```python
from build123d import *

# Parameters (mm, degrees)
F1_DEPTH  = 16
F2_W      = 70
F2_H      = 3
F3_DEPTH  = 2
F4_W      = 50
F4_H      = 12
F5_DEPTH  = 2
F6_R      = 1
F9_DEPTH  = 2
F11_DEPTH = 38.001
F13_D     = 4
F14_R     = 3
F14_R_2   = 2
F15_DEPTH = 5


with BuildPart() as f1:
    # F0 (on Front) → F1 (new body)
    with BuildSketch(Plane.XZ):
        with BuildLine():
            Line((46.2855722755, 5.7414249778), (-47.7144277245, 5.7414249778))
            ThreePointArc((-47.7144277245, 5.7414249778), (-58.7144277245, -5.2585750222), (-47.7144277245, -16.2585750222))
            Line((-47.7144277245, -16.2585750222), (-28.7144277245, -16.2585750222))
            ThreePointArc((-28.7144277245, -16.2585750222), (-25.7968307423, -17.5210599177), (-24.7197856057, -20.5120821569))
            ThreePointArc((-24.7197856057, -20.5120821569), (-0.5386319719, -49.8206199667), (35.0020481502, -63.2585750222))
            ThreePointArc((35.0020481502, -63.2585750222), (39.8678360266, -64.6074545818), (44.1721712505, -67.2471640366))
            Line((44.1721712505, -67.2471640366), (45.9107602648, -66.2585750222))
            ThreePointArc((45.9107602648, -66.2585750222), (40.9429054682, -62.6971545828), (35.0020481502, -61.2585750222))
            ThreePointArc((35.0020481502, -61.2585750222), (0.6230450398, -48.7022972109), (-22.7197856057, -20.5120821569))
            ThreePointArc((-22.7197856057, -20.5120821569), (-24.3830859689, -16.1065299122), (-28.7144277245, -14.2585750222))
            Line((-28.7144277245, -14.2585750222), (-47.7144277245, -14.2585750222))
            ThreePointArc((-47.7144277245, -14.2585750222), (-56.7144277245, -5.2585750222), (-47.7144277245, 3.7414249778))
            Line((-47.7144277245, 3.7414249778), (46.2855722755, 3.7414249778))
            Line((46.2855722755, 3.7414249778), (46.2855722755, 5.7414249778))
        make_face()
    extrude(amount=F1_DEPTH)

    # F2 (on face) → F3 (join)
    with BuildSketch(Plane.XY.offset(5.7414249778)):
        with Locations((11.2855722755, -17.5)):
            Rectangle(F2_W, F2_H)
    extrude(amount=-F3_DEPTH)

    # F4 (on face) → F5 (join)
    with BuildSketch(Plane.XZ.offset(19)):
        with Locations((21.2855722755, -2.2585750222)):
            Rectangle(F4_W, F4_H)
    extrude(amount=-F5_DEPTH)

    # F6
    f6_edges = [f1.edges().sort_by_distance(p)[0] for p in [
        (11.285572, -19, 5.741425),
        (21.285572, -17, 3.741425),
    ]]
    fillet(f6_edges, radius=F6_R)

    # F7: F1 across plane


with BuildPart() as f1_1:
    add(f1.part)
    add(f1.part.mirror(Plane.XZ))

    # F8 (on face) → F9 (cut)
    with BuildSketch(Plane.XY.offset(5.7414249778)):
        with BuildLine():
            Line((46.2855722755, 12), (-13.7144277245, 12))
            ThreePointArc((-13.7144277245, 12), (-25.7144277245, 0), (-13.7144277245, -12))
            Line((-13.7144277245, -12), (46.2855722755, -12))
            Line((46.2855722755, -12), (46.2855722755, 12))
        make_face()
    extrude(amount=-F9_DEPTH, mode=Mode.SUBTRACT)

    # F10 (on face) → F11 (cut, through all)
    with BuildSketch(Plane.XZ.offset(19)):
        with BuildLine():
            ThreePointArc((2.2855722755, -0.2585750222), (-0.7144277245, -3.2585750222), (2.2855722755, -6.2585750222))
            Line((2.2855722755, -6.2585750222), (22.2855722755, -6.2585750222))
            ThreePointArc((22.2855722755, -6.2585750222), (25.2855722755, -3.2585750222), (22.2855722755, -0.2585750222))
            Line((22.2855722755, -0.2585750222), (2.2855722755, -0.2585750222))
        make_face()
    extrude(amount=-F11_DEPTH, mode=Mode.SUBTRACT)

    # F13 (through all)
    with Locations(Plane.XZ.offset(19)):
        with Locations((32.2855722755, -2.2585750222)):
            Hole(F13_D / 2)

    # F14 (on face) → F15 (join)
    with BuildSketch(Plane(origin=(0, -17, 0), x_dir=(-1, 0, 0), z_dir=(0, 1, 0))):
        with Locations((-32.2855722755, -2.2585750222)):
            Circle(F14_R)
        with Locations((-32.2855722755, -2.2585750222)):
            Circle(F14_R_2, mode=Mode.SUBTRACT)
    extrude(amount=F15_DEPTH)


solid = f1_1.part
```
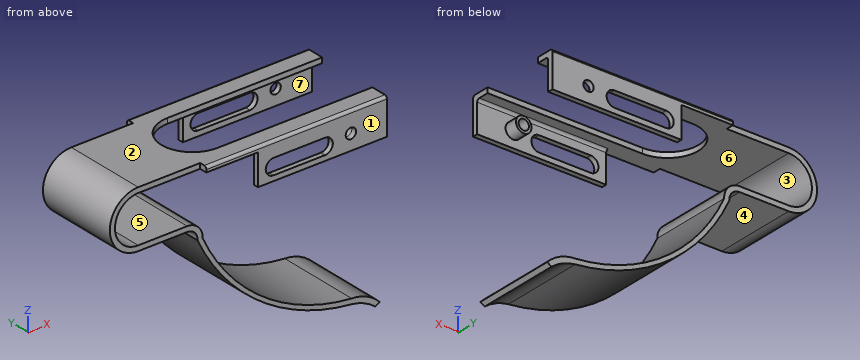
Design review of the part built by this model. Coordinates are the model's own, in mm. Face numbers are marked on the shaded views. A direction names the side the tool comes from. Round coordinates to 2 decimals unless told otherwise and drop trailing zeros. Write each loop counter-clockwise with the first axis right and the second up, starting at its lowest first coordinate (ties: lowest second). Pieces come first, ordered by that corner, then holes.
Item 1: For the marked faces 4, 5, 6 and 7, list the 3-axis set-ups (+Z, -Z, +X, -X, +Y, -Y) from which the entire face can be reached by the end or side of a thin tool; tool diameter is ignored.
Item 2: We need section D-D on z = -53.5. Write out the cut boundary in (x, y), and give its area (3 significant figures).
Item 3: We need section B-B on y = 0. Write out the cut boundary in (x, z).
Item 4: The part is to be moulded in two halves that separate along Z. For the marked faces 1, 2 and 3, say which applies: +Z half, -Z half, draft (parallel to the pull), parting line (faces both ways), or undercut.
Item 5: For probe 1 along X at (y, z) = (-13, -3); probe 2 along Z at (x, y) = (-53.5, -14.5); probe 3 along X at (y, z) = (2, -29.5), list the stretches that pass through material, from the lowest coordinate up.
Item 6: We need section A-A on x = -2.5. Write out the cut boundary in (y, z), and give its area (3 significant figures).
Item 7: Clearance check with flat-ended pins moving along their axes: pin 1 Ø1.6 at (x, y) = (10, 18) entering from -Z; pin 2 Ø0.6 at (y, z) = (17.5, 4.5) entering from -X; pin 3 Ø3 at (y, z) = (4.5, -49) entering from -X; pin 4 Ø3 at (x, z) = (32.29, -2.26) entering from -Y. State where each tip first meets the part, or that it passes through.
Item 8: We need section C-C on x = 24. Write out the cut boundary in (y, z), and give its area (3 significant figures).
Returned:
1. face 4: -Z, -X, +Y, -Y
1. face 5: +X, +Y, -Y
1. face 6: none
1. face 7: -Z, +X, -X
2. outline: (5.13, -16) - (8.47, -16) - (8.47, 16) - (5.13, 16) - close
2. area: 107 mm2
3. outline: (-47.71, -16.26) - (-28.71, -16.26) arc R4 cw to (-24.72, -20.51) arc R73.97 ccw to (35, -63.26) arc R18.11 cw to (44.17, -67.25) - (45.91, -66.26) arc R16 ccw to (35, -61.26) arc R70 cw to (-22.72, -20.51) arc R6 ccw to (-28.71, -14.26) - (-47.71, -14.26) arc R9 cw to (-47.71, 3.74) - (-25.71, 3.74) - (-25.71, 5.74) - (-47.71, 5.74) arc R11 ccw to start
4. face 1: draft
4. face 2: +Z half
4. face 3: undercut
5. probe 1: x = -58.48 to -56.43, 29.38 to 30.43, 34.14 to 35.19
5. probe 2: z = -14.61 to -12.15, 1.64 to 4.1
5. probe 3: x = -19.82 to -17.81
6. outline: (-19, -8.26) - (-17, -8.26) - (-17, 2.74) arc R1 cw to (-16, 3.74) - (-12, 3.74) - (-12, 5.74) - (-18, 5.74) arc R1 ccw to (-19, 4.74) - close; (-16, -48.37) - (16, -48.37) - (16, -46.36) - (-16, -46.36) - close; (12, 3.74) - (16, 3.74) arc R1 cw to (17, 2.74) - (17, -8.26) - (19, -8.26) - (19, 4.74) arc R1 ccw to (18, 5.74) - (12, 5.74) - close
6. area: 140 mm2
7. pin 1: stops at z = -8.26
7. pin 2: stops at x = -23.71
7. pin 3: stops at x = -3.61
7. pin 4: passes through
8. outline: (-19, -8.26) - (-17, -8.26) - (-17, -5.72) - (-19, -5.72) - close; (-19, -0.8) - (-17, -0.8) - (-17, 2.74) arc R1 cw to (-16, 3.74) - (-12, 3.74) - (-12, 5.74) - (-18, 5.74) arc R1 ccw to (-19, 4.74) - close; (-16, -61.29) - (16, -61.29) - (16, -59.42) - (-16, -59.42) - close; (12, 3.74) - (16, 3.74) arc R1 cw to (17, 2.74) - (17, -0.8) - (19, -0.8) - (19, 4.74) arc R1 ccw to (18, 5.74) - (12, 5.74) - close; (17, -8.26) - (19, -8.26) - (19, -5.72) - (17, -5.72) - close
8. area: 116 mm2
